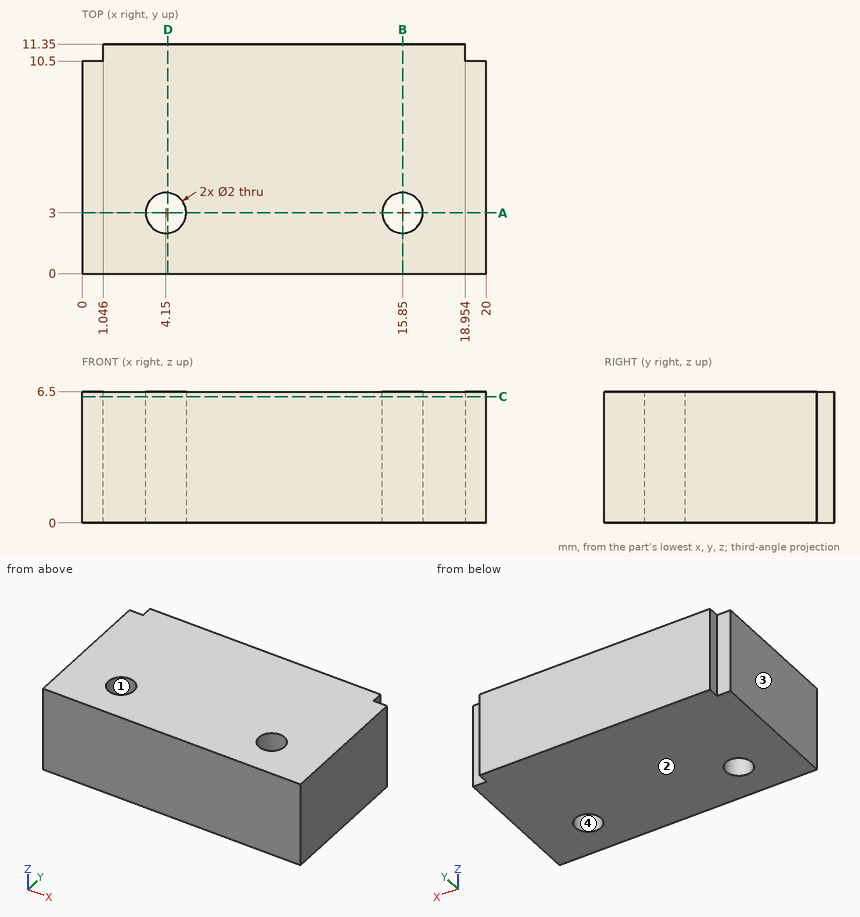
Study the drawing (mm; zero at the part's minimum x, y, z) and answer. Coordinates: 2 decimals unless noted, no trailing zeros. Loops run counter-clockwise (first coordinate to the right, second up) from the corner with the lowest first, then second, coordinate; pieces in that order, holes last. Notation, with made-up numbers: (-15, -29.75) -> (35, -29.75) arc R12 ccw to (35, -18.75) -> close; hole circle Ø11 at (70, -17). An arc over 180 degrees is marked (long way). Answer in a Markdown table with one row per item. Add a question column.
1. The part is cut by section C-C, the plane z = 6.25. Write down the section's boundary in (x, y), then the cut area to 3 significant figures.
2. Flat-ended cylindrical pins translate along their axes: P1, Ø3, axis at x = 4.15, y = 3, coming from the -Z side; P2, Ø0.8, axis at x = 19.5, z = 4.5, coming from the +Y side; P3, Ø0.7, axis at y = 11, z = 2, coming from the -X side; P4, Ø0.7, axis at y = 11, z = 4.5, coming from the +X side. Find the tip coordinate at first contact, or state that the pin passes through.
3. Determine the mould class of the marked faces 1, 2, 3 and 4 for opening direction X: +X half, -X half, draft (parallel to the pull), parting line (faces both ways), or undercut.
4. The part is cut by section A-A, the plane y = 3. Write down the section's boundary in (x, z).
5. Consider line 1 (Y direction, x = 4.15, z = 3); line 2 (X direction, y = 3.5, z = 1.25); line 3 (Y direction, x = 3.5, z = 1). Determine where each line is inside the solid, lowest interval first. Write a range as [from, to].
6. The part is cut by section D-D, the plane x = 4.25. Write down the section's boundary in (y, z) (3 decimals), then the cut area to 3 significant figures.
7. The part is cut by section B-B, the plane x = 15.85. Write down the section's boundary in (y, z), then the cut area to 3 significant figures.
Answer below:
| question | item | result |
|---|---|---|
| 1 | outline | (0, 0) -> (20, 0) -> (20, 10.5) -> (18.95, 10.5) -> (18.95, 11.35) -> (1.05, 11.35) -> (1.05, 10.5) -> (0, 10.5) -> close; hole circle Ø2 at (4.15, 3); hole circle Ø2 at (15.85, 3) |
| 1 | area | 219 mm2 |
| 2 | P1 | z = 0 |
| 2 | P2 | y = 10.5 |
| 2 | P3 | x = 1.05 |
| 2 | P4 | x = 18.95 |
| 3 | face 1 | undercut |
| 3 | face 2 | draft |
| 3 | face 3 | -X half |
| 3 | face 4 | undercut |
| 4 | outline | (0, 0) -> (3.15, 0) -> (3.15, 6.5) -> (0, 6.5) -> close; (5.15, 0) -> (14.85, 0) -> (14.85, 6.5) -> (5.15, 6.5) -> close; (16.85, 0) -> (20, 0) -> (20, 6.5) -> (16.85, 6.5) -> close |
| 5 | line 1 | [0, 2], [4, 11.35] |
| 5 | line 2 | [0, 3.28], [5.02, 14.98], [16.72, 20] |
| 5 | line 3 | [0, 2.24], [3.76, 11.35] |
| 6 | outline | (0, 0) -> (2.005, 0) -> (2.005, 6.5) -> (0, 6.5) -> close; (3.995, 0) -> (11.35, 0) -> (11.35, 6.5) -> (3.995, 6.5) -> close |
| 6 | area | 60.8 mm2 |
| 7 | outline | (0, 0) -> (2, 0) -> (2, 6.5) -> (0, 6.5) -> close; (4, 0) -> (11.35, 0) -> (11.35, 6.5) -> (4, 6.5) -> close |
| 7 | area | 60.8 mm2 |
